Could you check a few things on this model? Use its own coordinates, in mm. Face numbers are marked on the shaded views. A direction names the side the tool comes from. Give positions to 0.01 mm unless a question says otherwise; leave off trailing zeros. Loops run counter-clockwise (first coordinate to the right, second up) from the corner with the lowest first, then second, coordinate; pieces in that order, holes last. Notation, with made-up numbers: (11.5, 11) - (68.5, 11) arc R21 cw to (68.5, 17) - close; hole circle Ø8 at (31, -34.75). An arc over 180 degrees is marked (long way). One line per item, written item: value. Start each with the question number.
Q1. I want a section at B-B (y = -2). Please give me the cut outline in (x, z).
Q2. If I drill on line 1 (Y direction, x = 11, z = -3.5); line 2 (X direction, y = 0.25, z = -20); line 3 (Y direction, x = 8, z = -14.75) (1 decimal), over which ranges is the centre line in solid material (lowest first)? Write a range as from..to.
Q3. I want a section at C-C (z = -3.5). Please give me the cut outline in (x, y), then the cut area to 3 significant figures.
Q4. I'm going to push flat-ended pins straight in: P1, Ø1.5, axis at y = -3.5, z = -17.5, coming from the +X side; P2, Ø1, axis at y = -0.5, z = -3.5, coming from the -X side; P3, Ø1.1, axis at y = 0.5, z = -4, coming from the +X side. Where does each tip first touch, or does it pass through?
Q5. If we mould it in two halves opening along Y, with no side actions, what happens to the marked faces 1, 2 and 3? For each: released by +Y, released by -Y, zero draft, split by the parting line, or undercut.
Q6. I want a section at A-A (x = 21). Please give me the cut outline in (y, z), then the cut area to 3 significant figures.
Q7. For the marked faces 4, 5 and 6, which set-ups out of +Z, -Z, +X, -X, +Y, -Y let a thin tool reach every point of the face, with its end or its side?
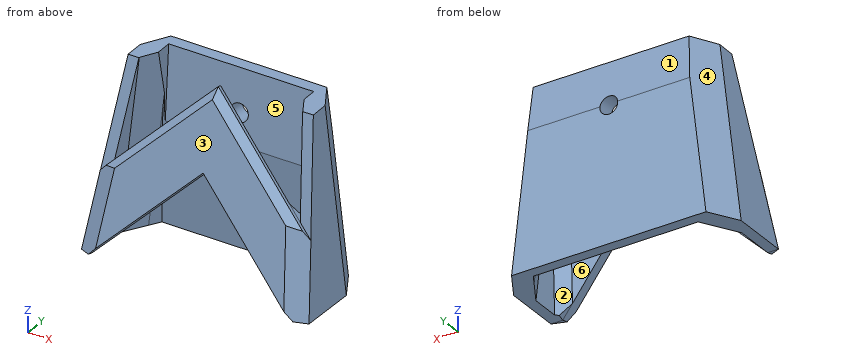
```python
from build123d import *
from OCP.BRepFilletAPI import BRepFilletAPI_MakeChamfer

# Parameters (mm, degrees)
EXTRUDE_3_DEPTH                  = 3
EXTRUDE_4_DEPTH                  = 12.5
CHAMFER_3_SIZE                   = 2
CHAMFER_3_SIZE2                  = 3.464101615
CHAMFER_4_SIZE                   = 4
CHAMFER_4_SIZE2                  = 2.309401077
CUT_EXTRUDE_2_DEPTH              = 41.277164746
CUT_EXTRUDE_2_DEPTH_BACK         = 41.277164746
EXTRUDE_5_DEPTH                  = 1.5
CUT_EXTRUDE_5_DEPTH              = 1.5
CHAMFER_7_SIZE                   = 1.5
CHAMFER_7_SIZE_2                 = 1.539926414
CHAMFER_8_SIZE                   = 2.598076211
CHAMFER_8_SIZE_2                 = 1.5
CHAMFER_10_SIZE                  = 1
CUT_EXTRUDE_START                = 2.76887
CUT_EXTRUDE_13_DEPTH             = 20.4
SKETCH_16_R                      = 1.25
CUT_EXTRUDE_14_DEPTH             = 10
CUT_EXTRUDE_15_REACH             = 54.631
CUT_EXTRUDE_START_2              = 13
CUT_EXTRUDE_15_DIRECTION_2_REACH = 54.631
CUT_EXTRUDE_START_3              = -5
CUT_EXTRUDE_16_DEPTH             = 45.631175115


# Some blends are built 0.0001 mm under size
with BuildPart() as part:
    # Эскиз5 → Бобышка-Вытянуть3 (new body)
    with BuildSketch(Plane(origin=(0, 0, 0), x_dir=(1, 0, 0), z_dir=(0, 1, 0))):
        Polygon((0, 0), (26, 0), (29, 25), (13, 25), (-3, 25), align=None)
    extrude(amount=EXTRUDE_3_DEPTH)

    # Эскиз6 → Бобышка-Вытянуть4 (add)
    with BuildSketch(Plane(origin=(0, 0, 0), x_dir=(-1, 0, 0), z_dir=(0, -1, 0))):
        Polygon((0, 0), (3, 25), (1.483218869, 25), (-1.516781131, 0), align=None)
        Polygon((-27.483218869, 25), (-29, 25), (-26, 0), (-24.483218869, 0), align=None)
    extrude(amount=EXTRUDE_4_DEPTH)

    # Фаска3
    chamfer_3_edges = [part.edges().sort_by_distance(p)[0] for p in [
        (0.016781131, 0, -12.5),
        (25.983218869, 0, -12.5),
    ]]
    chamfer_3_side = [part.faces().sort_by_distance(p)[0] for p in [
        (13, 0, -12.981390637),
    ]]
    chamfer(chamfer_3_edges, length=CHAMFER_3_SIZE, length2=CHAMFER_3_SIZE2, reference=chamfer_3_side[0])

    # Фаска4: one chamfer whose edges measure the first distance from different faces: ONE call of the kernel's chamfer builder (chamfer() names one face for all edges)
    chamfer_4_edges_1 = [part.edges().sort_by_distance(p)[0] for p in [
        (27.5, 3, -12.5),
    ]]
    chamfer_4_side_1 = [part.faces().sort_by_distance(p)[0] for p in [
        (27.5, -4.75, -12.5),
    ]]
    chamfer_4_edges_2 = [part.edges().sort_by_distance(p)[0] for p in [
        (-1.5, 3, -12.5),
    ]]
    chamfer_4_side_2 = [part.faces().sort_by_distance(p)[0] for p in [
        (-1.5, -4.75, -12.5),
    ]]
    chamfer_4 = BRepFilletAPI_MakeChamfer(part.part.solid().wrapped)
    for e in chamfer_4_edges_1:
        chamfer_4.Add(CHAMFER_4_SIZE, CHAMFER_4_SIZE2, e.wrapped, chamfer_4_side_1[0].wrapped)  # the first distance lies on this face
    for e in chamfer_4_edges_2:
        chamfer_4.Add(CHAMFER_4_SIZE, CHAMFER_4_SIZE2, e.wrapped, chamfer_4_side_2[0].wrapped)  # the first distance lies on this face
    add(Compound.cast(chamfer_4.Shape()), mode=Mode.REPLACE)

    # Эскиз7 → Вырез-Вытянуть2 (cut, two sides: drawn at the far end of the back side and taken through both)
    with BuildSketch(Plane(origin=(0, 0, 0), x_dir=(0, 0, -1), z_dir=(1, 0, 0)).offset(-CUT_EXTRUDE_2_DEPTH_BACK)):
        Polygon((25, -14), (25, -9), (0, -3.5), (0, -11), (0, -14), align=None)
    extrude(amount=CUT_EXTRUDE_2_DEPTH + CUT_EXTRUDE_2_DEPTH_BACK, mode=Mode.SUBTRACT)

    # Эскиз8 → Бобышка-Вытянуть5 (add)
    with BuildSketch(Plane(origin=(0, -3.33842045, 0.734452499), x_dir=(-1, 0, 0), z_dir=(0, -0.97664446670509, 0.2148617826751198))):
        Polygon((-29, 26.349867712), (3, 26.349867712), (0, 0.214861783), (-26, 0.214861783), align=None)
    extrude(amount=EXTRUDE_5_DEPTH)

    # Эскиз12 → Вырез-Вытянуть5 (cut)
    with BuildSketch(Plane(origin=(0, -4.80338715, 1.056745173), x_dir=(-1, 0, 0), z_dir=(0, -0.9766444667050901, 0.21486178267511977))):
        Polygon((-27.335370868, 26.349867712), (-13, 11.718369714), (1.483218869, 26.349867712), align=None)
        Polygon((-26, 0.214861783), (-13, 0.214861783), (-13, 1.069133834), (-27.836275269, 16.211883463), (-27.726463854, 15.255242802), align=None)
        Polygon((-13, 1.069133834), (-13, 0.214861783), (0, 0.214861783), (1.726463854, 15.255242802), (1.81620359, 16.037025649), align=None)
    extrude(amount=-CUT_EXTRUDE_5_DEPTH, mode=Mode.SUBTRACT)

    # Фаска7
    # the kernel refuses this chamfer: 1.539926414, 1.5 mm, written as the material it adds along each edge
    with BuildSketch(Plane(origin=(25.624388162, -5.592143703, -9.509744106), x_dir=(0.053421240321816, 0.9765759265760705, -0.20843615500811763), z_dir=(0.11640066814175269, -0.21340122492654667, -0.9700055678479392))) as chamfer_7_piece_1_section:
        Polygon((CHAMFER_7_SIZE * 0.99960211638, -CHAMFER_7_SIZE * 0.0282065405255), (-CHAMFER_7_SIZE_2 * 0.0537868652542, -CHAMFER_7_SIZE_2 * 0.998552439015), (0, 0), align=None)
    chamfer_7_piece_1 = extrude(amount=19.932121115, mode=Mode.PRIVATE)
    chamfer_7_piece_1 = split(chamfer_7_piece_1, bisect_by=Plane(origin=(26.215798587, -7.11837448, -25), z_dir=(0, 0, 1)), keep=Keep.TOP, mode=Mode.PRIVATE)
    chamfer_7_piece_1 = split(chamfer_7_piece_1, bisect_by=Plane(origin=(28.863675649, -6.560961429, -16.229864216), z_dir=(-0.7142981809435934, -0.1503691897591953, -0.6834963170872516)), keep=Keep.TOP, mode=Mode.PRIVATE)
    chamfer_7_piece_1 = split(chamfer_7_piece_1, bisect_by=Plane(origin=(23.540170532, -7.681629481, -21.323809907), z_dir=(0.7142981809435934, 0.15036918975919533, 0.6834963170872517)), keep=Keep.TOP, mode=Mode.PRIVATE)
    add(chamfer_7_piece_1)

    # Фаска8
    chamfer_8_edges_1 = [part.edges().sort_by_distance(p)[0] for p in [
        (-2.408101795, -9.357048885, -19.641717258),
    ]]
    chamfer_8_side_1 = [part.faces().sort_by_distance(p)[0] for p in [
        (-2.378297509, -9.357783968, -19.645058546),
    ]]
    chamfer_8_edges_2 = [part.edges().sort_by_distance(p)[0] for p in [
        (28.418137634, -9.375834016, -19.727104216),
    ]]
    chamfer_8_side_2 = [part.faces().sort_by_distance(p)[0] for p in [
        (28.388333349, -9.376569099, -19.730445503),
    ]]
    chamfer_8 = BRepFilletAPI_MakeChamfer(part.part.solid().wrapped)
    for e in chamfer_8_edges_1:
        chamfer_8.Add(CHAMFER_8_SIZE - 0.0001, CHAMFER_8_SIZE_2 - 0.0001, e.wrapped, chamfer_8_side_1[0].wrapped)
    for e in chamfer_8_edges_2:
        chamfer_8.Add(CHAMFER_8_SIZE - 0.0001, CHAMFER_8_SIZE_2 - 0.0001, e.wrapped, chamfer_8_side_2[0].wrapped)
    add(Compound.cast(chamfer_8.Shape()), mode=Mode.REPLACE)  # a hair under: the kernel refuses the full size

    # Фаска10
    chamfer_10_edges = [part.edges().sort_by_distance(p)[0] for p in [
        (7.070930475, -6.320076094, -5.837295478),
        (18.937101702, -6.335110761, -5.905634875),
    ]]
    chamfer(chamfer_10_edges, length=CHAMFER_10_SIZE)

    # Эскиз15 → Вырез-Вытянуть13 (cut)
    with BuildSketch(Plane(origin=(0, 0, 0), x_dir=(0, 0, -1), z_dir=(1, 0, 0)).offset(CUT_EXTRUDE_START)):
        Polygon((-0.003394727, -2.1), (12.496605273, -2.1), (12.496605273, 0), (-0.003394727, 0.9), align=None)
    extrude(amount=CUT_EXTRUDE_13_DEPTH, mode=Mode.SUBTRACT)

    # Эскиз16 → Вырез-Вытянуть14 (cut)
    with BuildSketch(Plane(origin=(0, 0.891145714, -0.119581473), x_dir=(-1, 0, 0), z_dir=(0, -0.9974180343569141, 0.0718140984736978))):
        with Locations(Location((-13, 5.84494773, 0), (0, 0, 90))):
            Circle(SKETCH_16_R)
    extrude(amount=-CUT_EXTRUDE_14_DEPTH, mode=Mode.SUBTRACT)

    # Вырез-Вытянуть15: up to this plane
    cut_extrude_15_end = Plane(origin=(1.516781131, -3.464101615, 0), z_dir=(0.8598565649588564, -0.4999999999999951, -0.10318278779506272))
    # Эскиз17 → Вырез-Вытянуть15 (cut, up to the surface)
    with BuildSketch(Plane(origin=(0, 0, 0), x_dir=(0, 0, -1), z_dir=(1, 0, 0)).offset(CUT_EXTRUDE_START_2), mode=Mode.PRIVATE) as cut_extrude_15_sk1:
        Polygon((25, 1.5), (8.333333333, 0), (8.333333333, -2.621768853), (25, -2.621768853), align=None)
    cut_extrude_15_tool1 = split(extrude(cut_extrude_15_sk1.sketch, amount=-CUT_EXTRUDE_15_REACH, mode=Mode.PRIVATE), bisect_by=cut_extrude_15_end, keep=Keep.BOTH, mode=Mode.PRIVATE)
    add(cut_extrude_15_tool1.solids().sort_by_distance((13, -0.90808, -17.284542))[0], mode=Mode.SUBTRACT)

    # Вырез-Вытянуть15 direction 2: up to this plane
    cut_extrude_15_direction_2_end = Plane(origin=(24.483218869, -3.464101615, 0), z_dir=(-0.859856564958857, -0.49999999999999406, -0.10318278779506279))
    # Эскиз17 → Вырез-Вытянуть15 direction 2 (cut, up to the surface)
    with BuildSketch(Plane(origin=(0, 0, 0), x_dir=(0, 0, -1), z_dir=(1, 0, 0)).offset(CUT_EXTRUDE_START_2), mode=Mode.PRIVATE) as cut_extrude_15_direction_2_sk1:
        Polygon((25, 1.5), (8.333333333, 0), (8.333333333, -2.621768853), (25, -2.621768853), align=None)
    cut_extrude_15_direction_2_tool1 = split(extrude(cut_extrude_15_direction_2_sk1.sketch, amount=CUT_EXTRUDE_15_DIRECTION_2_REACH, mode=Mode.PRIVATE), bisect_by=cut_extrude_15_direction_2_end, keep=Keep.BOTH, mode=Mode.PRIVATE)
    add(cut_extrude_15_direction_2_tool1.solids().sort_by_distance((13, -0.90808, -17.284542))[0], mode=Mode.SUBTRACT)

    # Эскиз18 → Вырез-Вытянуть16 (cut, through all)
    with BuildSketch(Plane(origin=(0, 0, 0), x_dir=(0, 0, -1), z_dir=(1, 0, 0)).offset(CUT_EXTRUDE_START_3)):
        Polygon((6, 3), (0, 2.5), (0, 3), align=None)
        Polygon((0.202280253, -4.056458685), (0, 2.5), (0, -4.056458685), align=None)
    extrude(amount=CUT_EXTRUDE_16_DEPTH, mode=Mode.SUBTRACT)


solid = part.part
```
Worked answers:
1. outline: (-3, -25) - (-0.63, -25) - (2.35, -0.14) - (-0.02, -0.14) - close; (23.65, -0.14) - (26.63, -25) - (29, -25) - (26.02, -0.14) - close
2. line 1: y = -5.81..-4.27, 0.65..2.79
2. line 2: x = -1.67..1.28, 24.72..27.67
2. line 3: y = -8.3..-6.7, 0.6..3
3. outline: (-0.42, -4.27) - (1.1, -4.27) - (1.1, -3.46) - (2.77, -0.59) - (2.77, 0.65) - (23.17, 0.65) - (23.17, -0.48) - (24.9, -3.46) - (24.9, -4.27) - (26.42, -4.27) - (26.42, -1) - (24.22, 2.79) - (1.78, 2.79) - (-0.42, -1) - close; (9.66, -4.78) - (10.85, -5.81) - (15.12, -5.81) - (16.31, -4.78) - (16.2, -4.27) - (9.77, -4.27) - close
3. area: 82.1 mm²
4. P1: stops at x = 28.19
4. P2: stops at x = -0.43
4. P3: stops at x = 25.93
5. face 1: released by +Y
5. face 2: undercut
5. face 3: released by -Y
6. outline: (-9.08, -18.36) - (-7.61, -18.68) - (-5.32, -8.28) - (-5.81, -8.18) - (-7.09, -9.36) - close; (0.17, -10.18) - (1.5, -25) - (3, -25) - (3, -6) - (2.5, 0) - (0.9, -0.05) - close
6. area: 70.9 mm²
7. face 4: +Z, -X, +Y
7. face 5: +Z
7. face 6: -Z
